Job drawing, mm, ordinate dimensions from the low corner. One solid piece. A direction names the side the tool comes from. Round coordinates to 2 decimals unless told otherwise and drop trailing zeros. Loops run counter-clockwise (first coordinate to the right, second up) from the corner with the lowest first, then second, coordinate; pieces in that order, holes last.
1) Mould opens along X. For the marked faces 1, 2 and 3 say: +X half, -X half, draft (parallel to the pull), parting line (faces both ways), or undercut.
2) Band-saw the part on A-A, the plane z = 4. Write the cut outline in (x, y).
3) Band-saw the part on B-B, the plane x = 11. Write the cut outline in (y, z), then the cut area to 3 significant figures.
4) Band-saw the part on D-D, the plane z = 6.75. Write the cut outline in (x, y), then the cut area to 3 significant figures.
5) 3-axis set-ups, long thin cutter, end or side, ignore diameter. For the marked faces 4, 5 and 6: which of +Z, -Z, +X, -X, +Y, -Y reach the whole face in a straight line?
6) Band-saw the part on C-C, the plane y = 4. Write the cut outline in (x, z).
7) Probe line 1 (X direction, y = 4.5, z = 5); line 2 (Z direction, x = 11, y = 3.85); line 3 (X direction, y = 0.5, z = 2.25). List the from-to ranges inside material, lowest first.
8) Drop flat-ended pins along their axis: P1, Ø3, axis at x = 12, z = 5.5, coming from the +Y side; P2, Ø1.5, axis at x = 14, z = 3, coming from the -Y side; P3, Ø4, axis at x = 10, y = 0.5, coming from the +Z side; P4, Ø0.6, axis at y = 5.5, z = 6.5, coming from the +X side. Give the stop position or say it passes through.
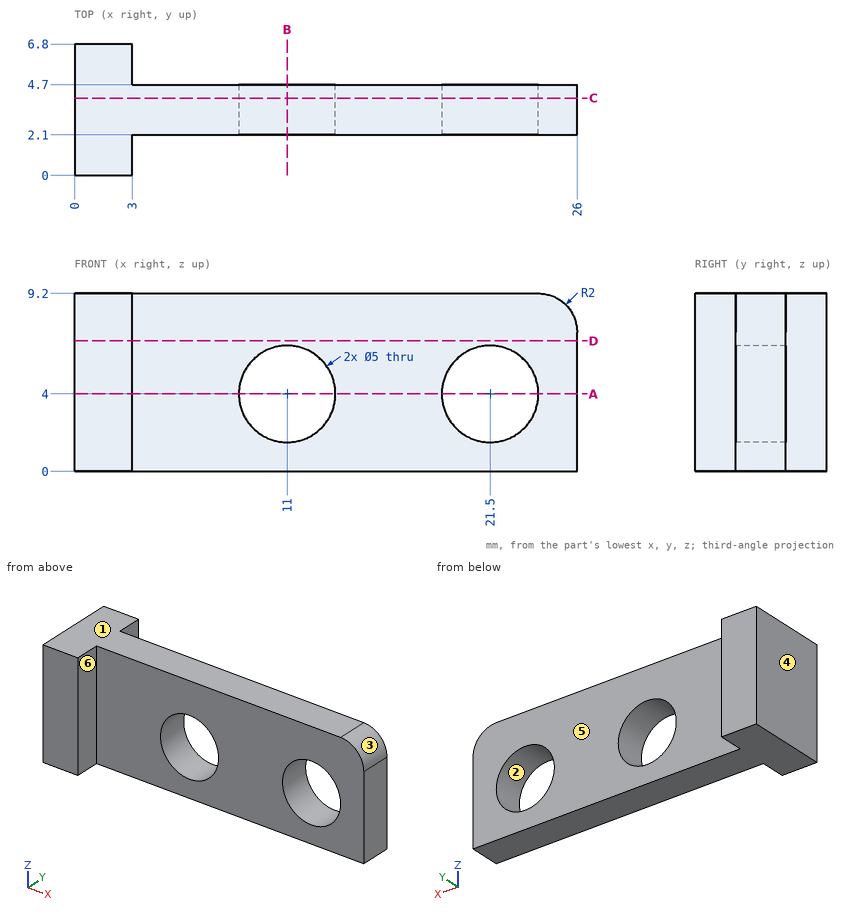
Reported:
1. face 1: draft
1. face 2: undercut
1. face 3: +X half
2. outline: (0, 0) - (3, 0) - (3, 2.1) - (8.5, 2.1) - (8.5, 4.7) - (3, 4.7) - (3, 6.8) - (0, 6.8) - close; (13.5, 2.1) - (19, 2.1) - (19, 4.7) - (13.5, 4.7) - close; (24, 2.1) - (26, 2.1) - (26, 4.7) - (24, 4.7) - close
3. outline: (2.1, 0) - (4.7, 0) - (4.7, 1.5) - (2.1, 1.5) - close; (2.1, 6.5) - (4.7, 6.5) - (4.7, 9.2) - (2.1, 9.2) - close
3. area: 10.9 mm2
4. outline: (0, 0) - (3, 0) - (3, 2.1) - (26, 2.1) - (26, 4.7) - (3, 4.7) - (3, 6.8) - (0, 6.8) - close
4. area: 80.2 mm2
5. face 4: +Z, -Z, -X, +Y, -Y
5. face 5: +Z, -Z, +X, +Y
5. face 6: +Z, -Z, +X, -Y
6. outline: (0, 0) - (26, 0) - (26, 7.2) arc R2 ccw to (24, 9.2) - (0, 9.2) - close; hole circle Ø5 at (11, 4); hole circle Ø5 at (21.5, 4)
7. line 1: x = 0 to 8.71, 13.29 to 19.21, 23.79 to 26
7. line 2: z = 0 to 1.5, 6.5 to 9.2
7. line 3: x = 0 to 3
8. P1: stops at y = 4.7
8. P2: stops at y = 2.1
8. P3: stops at z = 9.2
8. P4: stops at x = 3
